The model under review builds one solid part; all positions refer to its coordinate system, in mm. A direction names the side the tool comes from. Round coordinates to 2 decimals unless told otherwise and drop trailing zeros. Order: outer loops, then holes, each group sorted by start corner. A loop starts at its lowest first (then second) coordinate and runs counter-clockwise, first axis right, second up.
```python
from build123d import *

# Parameters (mm, degrees)
SKETCH2_W           = 70
SKETCH2_H           = 40
BOSS_EXTRUDE1_DEPTH = 30
CUT_EXTRUDE2_DEPTH  = 49
SKETCH5_W           = 20
SKETCH5_H           = 10
CUT_EXTRUDE3_DEPTH  = 49
SKETCH6_W           = 40
SKETCH6_H           = 5
CUT_EXTRUDE4_DEPTH  = 30
SKETCH7_W           = 10
SKETCH7_H           = 5
CUT_EXTRUDE5_DEPTH  = 41
SKETCH8_R           = 5
CUT_EXTRUDE6_DEPTH  = 31
SKETCH9_R           = 5
CUT_EXTRUDE7_DEPTH  = 31


with BuildPart() as part:
    # Sketch2 → Boss-Extrude1 (new body)
    with BuildSketch(Plane(origin=(0, 0, 0), x_dir=(1, 0, 0), z_dir=(0, 1, 0))):
        with Locations((35, 20)):
            Rectangle(SKETCH2_W, SKETCH2_H)
    extrude(amount=BOSS_EXTRUDE1_DEPTH)

    # Sketch4 → Cut-Extrude2 (cut)
    with BuildSketch(Plane.XY):
        Polygon((70, 30), (30, 30), (70, 10), align=None)
    extrude(amount=-CUT_EXTRUDE2_DEPTH, mode=Mode.SUBTRACT)

    # Sketch5 → Cut-Extrude3 (cut)
    with BuildSketch(Plane(origin=(0, 0, 0), x_dir=(-1, 0, 0), z_dir=(0, -1, 0))):
        with Locations((-60, 5)):
            Rectangle(SKETCH5_W, SKETCH5_H)
    extrude(amount=-CUT_EXTRUDE3_DEPTH, mode=Mode.SUBTRACT)

    # Sketch6 → Cut-Extrude4 (cut)
    with BuildSketch(Plane.ZY):
        with Locations((-20, 2.5)):
            Rectangle(SKETCH6_W, SKETCH6_H)
    extrude(amount=-CUT_EXTRUDE4_DEPTH, mode=Mode.SUBTRACT)

    # Sketch7 → Cut-Extrude5 (cut, through all)
    with BuildSketch(Plane.ZY.offset(-30)):
        with Locations((-25, 2.5)):
            Rectangle(SKETCH7_W, SKETCH7_H)
    extrude(amount=-CUT_EXTRUDE5_DEPTH, mode=Mode.SUBTRACT)

    # Sketch8 → Cut-Extrude6 (cut, through all)
    with BuildSketch(Plane(origin=(0, 30, 0), x_dir=(1, 0, 0), z_dir=(0, 1, 0))):
        with Locations((10, 10)):
            Circle(SKETCH8_R)
    extrude(amount=-CUT_EXTRUDE6_DEPTH, mode=Mode.SUBTRACT)

    # Sketch9 → Cut-Extrude7 (cut, through all)
    with BuildSketch(Plane(origin=(0, 30, 0), x_dir=(1, 0, 0), z_dir=(0, 1, 0))):
        with Locations((20, 30)):
            Circle(SKETCH9_R)
    extrude(amount=-CUT_EXTRUDE7_DEPTH, mode=Mode.SUBTRACT)


solid = part.part
```
(1) To check wall thickness, follow probe 1 along Z at (x, y) = (20, 11.25); probe 2 along Z at (x, y) = (10, 16.5); probe 3 along Y at (x, z) = (4, -22). State the ranges of each line that lie inside material, in increasing order.
Data:
probe 1: z = -40 to -35, -25 to 0
probe 2: z = -40 to -15, -5 to 0
probe 3: y = 5 to 30
(2) Consider section C-C (x = 33). Write out the cut boundary in (y, z).
Data:
outline: (0, -40) - (28.5, -40) - (28.5, 0) - (0, 0) - (0, -20) - (5, -20) - (5, -30) - (0, -30) - close
(3) Insertion check: pin 1 (5.5 mm diameter, centred on x = 58, y = 2, fed in from +Z); pin 2 (12 mm diameter, centred on x = 36.5, z = -23, fed in from +Y); pin 3 (12 mm diameter, centred on y = 4, z = -23, fed in from +X); pin 4 (10 mm diameter, centred on x = 23.5, z = -13, fed in from -Y). Each pin has a flat end and moves straight along its axis. Give the tip position at first contact, or say it passes through.
Data:
pin 1: stops at z = -10
pin 2: stops at y = 29.75
pin 3: stops at x = 70
pin 4: stops at y = 5
(4) Consider section D-D (y = 6.75). Write out the cut boundary in (x, z), and give its area (3 significant figures).
Data:
outline: (0, -40) - (70, -40) - (70, -10) - (50, -10) - (50, 0) - (0, 0) - close; hole circle Ø10 at (10, -10); hole circle Ø10 at (20, -30)
area: 2,440 mm2
(5) Consider section B-B (x = 20). Write out the cut boundary in (y, z).
Data:
outline: (5, -40) - (30, -40) - (30, -35) - (5, -35) - close; (5, -25) - (30, -25) - (30, 0) - (5, 0) - close
(6) Draft analysis for pull direction X (two halves, no side actions). For faces 1 (the flat face through (45, 0, -12)), 2 (the cylindrical face through (14.77, 17.68, -11.5)), 3 (the flat face through (30, 3, -35)), state which applies: pulls with the +X half, pulls with the -X half, needs draft (parallel to the pull), parting line crosses it, or undercut.
Data:
face 1: needs draft
face 2: undercut
face 3: pulls with the -X half
(7) Consider section A-A (y = 11.5). Write out the cut boundary in (x, z).
Data:
outline: (0, -40) - (67, -40) - (67, -10) - (50, -10) - (50, 0) - (0, 0) - close; hole circle Ø10 at (10, -10); hole circle Ø10 at (20, -30)
(8) For faces 4 (the flat face through (60, 8, -10)), 5 (the flat face through (50, 2, -20)), 6 (the flat face through (30, 3, -10)), list the 3-axis set-ups (+Z, -Z, +X, -X, +Y, -Y) from which the entire face can be reached by the end or side of a thin tool; tool diameter is ignored.
Data:
face 4: +Z, +X, +Y, -Y
face 5: +X, -X, -Y
face 6: +Z, -Z, -X, -Y
